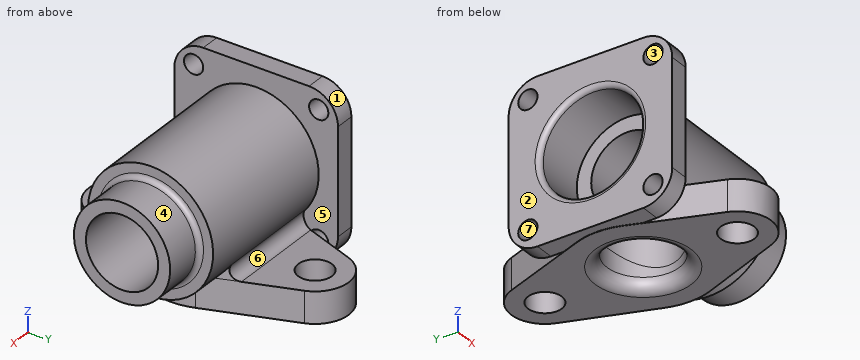
```python
from build123d import *

# Parameters (mm, degrees)
SKETCH1_R           = 7
SKETCH1_R_2         = 15
BOSS_EXTRUDE1_DEPTH = 13
SKETCH2_R           = 4
BOSS_EXTRUDE2_DEPTH = 4
SKETCH5_R           = 26
BOSS_EXTRUDE3_DEPTH = 63
FILLET6_R           = 4
FILLET7_R           = 4
SKETCH6_R           = 21
CUT_EXTRUDE1_DEPTH  = 22
CUT_EXTRUDE2_REACH  = 93.894
SKETCH7_R           = 15
BOSS_EXTRUDE4_START = -43
SKETCH9_R           = 15
BOSS_EXTRUDE4_DEPTH = 43
FILLET10_R          = 2
SKETCH12_R          = 20
BOSS_EXTRUDE5_DEPTH = 17
FILLET14_R          = 2
CUT_EXTRUDE4_REACH  = 119.421
SKETCH16_R          = 15
CUT_EXTRUDE5_REACH  = 106.103
SKETCH17_R          = 15
FILLET17_R          = 5


with BuildPart() as part:
    # Sketch1 → Boss-Extrude1 (new body)
    with BuildSketch(Plane.XY):
        with BuildLine():
            Line((-13.182592111, 45.551865312), (-26.129780791, 9.343289347))
            ThreePointArc((-26.129780791, 9.343289347), (-27.749182892, -0.212952692), (-25.983307196, -9.743215442))
            Line((-25.983307196, -9.743215442), (-13.108695522, -44.07736233))
            ThreePointArc((-13.108695522, -44.07736233), (0, -53.161866251), (13.108695522, -44.07736233))
            Line((13.108695522, -44.07736233), (25.983307196, -9.743215442))
            ThreePointArc((25.983307196, -9.743215442), (27.749182892, -0.212952692), (26.129780791, 9.343289347))
            Line((26.129780791, 9.343289347), (13.182592111, 45.551865312))
            ThreePointArc((13.182592111, 45.551865312), (0, 54.838133749), (-13.182592111, 45.551865312))
        make_face()
        with Locations((0, 40.838133749)):
            Circle(SKETCH1_R, mode=Mode.SUBTRACT)
        with Locations((0, -39.161866251)):
            Circle(SKETCH1_R, mode=Mode.SUBTRACT)
        Circle(SKETCH1_R_2, mode=Mode.SUBTRACT)
    extrude(amount=-BOSS_EXTRUDE1_DEPTH)



with BuildPart() as body_2:
    # Sketch2 → Boss-Extrude2 (new, symmetric)
    with BuildSketch(Plane(origin=(-27.5, 0, 0), x_dir=(0, 0, -1), z_dir=(1, 0, 0))):
        with BuildLine():
            Line((-43.103277086, 34), (0.896722914, 34))
            ThreePointArc((0.896722914, 34), (9.382004289, 30.485281374), (12.896722914, 22))
            Line((12.896722914, 22), (12.896722914, -22))
            ThreePointArc((12.896722914, -22), (9.382004289, -30.485281374), (0.896722914, -34))
            Line((0.896722914, -34), (-43.103277086, -34))
            ThreePointArc((-43.103277086, -34), (-51.58855846, -30.485281374), (-55.103277086, -22))
            Line((-55.103277086, -22), (-55.103277086, 22))
            ThreePointArc((-55.103277086, 22), (-51.58855846, 30.485281374), (-43.103277086, 34))
        make_face()
        with Locations((-47.103277086, 26)):
            Circle(SKETCH2_R, mode=Mode.SUBTRACT)
        with Locations((-47.103277086, -26)):
            Circle(SKETCH2_R, mode=Mode.SUBTRACT)
        with Locations((4.896722914, 26)):
            Circle(SKETCH2_R, mode=Mode.SUBTRACT)
        with Locations((4.896722914, -26)):
            Circle(SKETCH2_R, mode=Mode.SUBTRACT)
    extrude(amount=BOSS_EXTRUDE2_DEPTH, both=True)


with BuildPart() as part_1:
    add(part.part)

    add(body_2.part)  # Boss-Extrude3 merges body 2
    # Sketch5 → Boss-Extrude3 (add)
    with BuildSketch(Plane(origin=(-23.5, 0, 0), x_dir=(0, 0, -1), z_dir=(1, 0, 0))):
        with Locations(Location((-21.103277086, 0, 0), (0, 0, 324.258878137))):
            Circle(SKETCH5_R)
    extrude(amount=BOSS_EXTRUDE3_DEPTH)

    # Fillet6
    # the kernel refuses this fillet: 4 mm, written as the material it adds along each edge
    with BuildSketch(Plane(origin=(-47.149613866, -15.187221479, 0), x_dir=(0, -0.701013336910265, 0.7131481623575392), z_dir=(1, 0, 0))) as fillet6_piece_1_section:
        with BuildLine():
            CenterArc((9.484070542, 3.94221812), FILLET6_R, 135.491639194, 124.757843476)
            Line((6.631477893, 6.746271467), (0, 0))
            ThreePointArc((0, 0), (4.403318466, 0.375582222), (8.806636932, 0))
        make_face()
    fillet6_piece_1 = extrude(amount=94.74114261, mode=Mode.PRIVATE)
    fillet6_piece_1 = split(fillet6_piece_1, bisect_by=Plane(origin=(19.603312595, -26.757450692, 1.537679947), z_dir=(-0.9363353944532133, 0.35110686278417497, 0)), keep=Keep.TOP, mode=Mode.PRIVATE)
    fillet6_piece_1 = split(fillet6_piece_1, bisect_by=Plane(origin=(-19.602415947, -26.759841882, 1.537679947), z_dir=(0.9363353944532126, 0.35110686278417685, 0)), keep=Keep.TOP, mode=Mode.PRIVATE)
    add(fillet6_piece_1)

    # Fillet7
    # the kernel refuses this fillet: 4 mm, written as the material it adds along each edge
    with BuildSketch(Plane(origin=(47.689765613, 15.187221479, 0), x_dir=(0, 1, 0), z_dir=(-1, 0, 0))) as fillet7_piece_1_section:
        with BuildLine():
            CenterArc((9.459845546, -4), FILLET7_R, 90, 124.757843476)
            ThreePointArc((6.173569943, -6.280436945), (3.354630742, -2.876930326), (0, 0))
            Line((0, 0), (9.459845546, 0))
        make_face()
    fillet7_piece_1 = extrude(amount=94.839379478, mode=Mode.PRIVATE)
    fillet7_piece_1 = split(fillet7_piece_1, bisect_by=Plane(origin=(-19.975054308, 26.555819952, 1.538101515), z_dir=(0.941613722197052, -0.33669511159239174, 0)), keep=Keep.TOP, mode=Mode.PRIVATE)
    fillet7_piece_1 = split(fillet7_piece_1, bisect_by=Plane(origin=(19.97656332, 26.551599793, 1.538101515), z_dir=(-0.9416137221970524, -0.3366951115923907, 0)), keep=Keep.TOP, mode=Mode.PRIVATE)
    add(fillet7_piece_1)

    # Sketch6 → Cut-Extrude1 (cut)
    with BuildSketch(Plane.ZY.offset(31.5)):
        with Locations((21.103277086, 0)):
            Circle(SKETCH6_R)
    extrude(amount=-CUT_EXTRUDE1_DEPTH, mode=Mode.SUBTRACT)

    # Sketch7 → Cut-Extrude2 (cut, up to next)
    with BuildSketch(Plane.ZY.offset(9.5), mode=Mode.PRIVATE) as cut_extrude2_sk1:
        with Locations((21.103277086, 0)):
            Circle(SKETCH7_R)
    cut_extrude2_tool1 = extrude(cut_extrude2_sk1.sketch, amount=-CUT_EXTRUDE2_REACH, mode=Mode.PRIVATE) & part_1.part
    add(cut_extrude2_tool1.solids().sort_by_distance((-9.5, 0, 21.103277))[0], mode=Mode.SUBTRACT)

    # Sketch9 → Boss-Extrude4 (add)
    with BuildSketch(Plane(origin=(39.5, 0, 0), x_dir=(0, 0, -1), z_dir=(1, 0, 0)).offset(BOSS_EXTRUDE4_START)):
        with Locations(Location((-21.103277086, 0, 0), (0, 0, 180))):
            Circle(SKETCH9_R)
    extrude(amount=BOSS_EXTRUDE4_DEPTH)

    # Fillet10
    fillet10_edges = [part_1.edges().sort_by_distance(p)[0] for p in [
        (-31.5, 0, 0.103277086),
    ]]
    fillet(fillet10_edges, radius=FILLET10_R)

    # Sketch12 → Boss-Extrude5 (add)
    with BuildSketch(Plane(origin=(39.5, 0, 0), x_dir=(0, 0, -1), z_dir=(1, 0, 0))):
        with Locations((-21.103277086, 0)):
            Circle(SKETCH12_R)
    extrude(amount=BOSS_EXTRUDE5_DEPTH)

    # Fillet14
    fillet14_edges = [part_1.edges().sort_by_distance(p)[0] for p in [
        (39.5, 0, 41.103277086),
    ]]
    fillet(fillet14_edges, radius=FILLET14_R)

    # Sketch16 → Cut-Extrude4 (cut, up to next)
    with BuildSketch(Plane(origin=(56.5, 0, 0), x_dir=(0, 0, -1), z_dir=(1, 0, 0)), mode=Mode.PRIVATE) as cut_extrude4_sk1:
        with Locations(Location((-21.103277086, 0, 0), (0, 0, 180))):
            Circle(SKETCH16_R)
    cut_extrude4_tool1 = extrude(cut_extrude4_sk1.sketch, amount=-CUT_EXTRUDE4_REACH, mode=Mode.PRIVATE) & part_1.part
    add(cut_extrude4_tool1.solids().sort_by_distance((56.5, 0, 21.103277))[0], mode=Mode.SUBTRACT)

    # Sketch17 → Cut-Extrude5 (cut, up to next)
    with BuildSketch(Plane(origin=(0, 0, -13), x_dir=(-1, 0, 0), z_dir=(0, 0, -1)), mode=Mode.PRIVATE) as cut_extrude5_sk1:
        with Locations(Location((0, 0, 0), (0, 0, 180))):
            Circle(SKETCH17_R)
    cut_extrude5_tool1 = extrude(cut_extrude5_sk1.sketch, amount=-CUT_EXTRUDE5_REACH, mode=Mode.PRIVATE) & part_1.part
    add(cut_extrude5_tool1.solids().sort_by_distance((0, 0, -13))[0], mode=Mode.SUBTRACT)

    # Fillet17
    fillet17_edges = [part_1.edges().sort_by_distance(p)[0] for p in [
        (-15, 0, -13),
    ]]
    fillet(fillet17_edges, radius=FILLET17_R)


solid = part_1.part
```
For this review, take the finished solid that the model builds, in its own axes (mm). Face numbers are marked on the shaded views. A direction names the side the tool comes from. Coordinates: 2 decimals unless noted, no trailing zeros. Order: outer loops, then holes, each group sorted by start corner. A loop starts at its lowest first (then second) coordinate and runs counter-clockwise, first axis right, second up. Notation, with made-up numbers: (42, 67.25) - (101, 67.25) arc R21 cw to (101, 88.25) - close; hole circle Ø9 at (-9.75, 46.25). An arc over 180 degrees is marked (long way). Answer as a JSON object with one key per item and string values. Group by question number.
1. We need section A-A on y = 0. Give the number of separate pieces and of enclosed holes in the cut face, then the cut area to 3 significant figures.
2. The part is to be moulded in two halves that separate along Z. For the marked faces 1, 2, 3 and 4, say which applies: pulls with the +Z half, pulls with the -Z half, needs draft (parallel to the pull), parting line crosses it, or undercut.
3. We need section C-C on x = 0. State the section outline as (y, z) points, then the cut area to 3 significant figures.
4. For probe 1 along X at (y, z) = (0, -6); probe 2 along Z at (x, y) = (11, 27.5); probe 3 along X at (y, z) = (0, -4.25), list the stretches that pass through material, from the lowest coordinate up.
5. For the marked faces 5, 6 and 7, list the 3-axis set-ups (+Z, -Z, +X, -X, +Y, -Y) from which the entire face can be reached by the end or side of a thin tool; tool diameter is ignored.
6. We need section B-B on y = 28. State the section outline as (x, z) points.
7. Clearance check with flat-ended pins moving along their axes: P1, Ø8.5, axis at x = 0, y = 40.84, coming from the +Z side; P2, Ø14.5, axis at x = 9.5, y = -42, coming from the +Z side; P3, Ø10, axis at y = 6.5, z = 30, coming from the -X side; P4, Ø2.5, axis at x = -26.5, z = 26, coming from the -Y side. State where each tip first meets the part, or that it passes through.
Final values:
{
 "1": {"separate pieces": "3", "enclosed holes": "0", "area": "1,460 mm²"},
 "2": {"face 1": "pulls with the +Z half", "face 2": "needs draft", "face 3": "undercut", "face 4": "parting line crosses it"},
 "3": {"outline": "(-53.16, -13) - (-46.16, -13) - (-46.16, 0) - (-53.16, 0) - close; (-32.16, -13) - (-20, -13) arc R5 ccw to (-15, -8) - (-15, 21.1) arc R15 cw to (15, 21.1) - (15, -8) arc R5 ccw to (20, -13) - (33.84, -13) - (33.84, 0) - (24.65, 0) arc R4 cw to (21.36, 6.28) arc R26 ccw (long way) to (-21.36, 6.28) arc R4 cw to (-24.65, 0) - (-32.16, 0) - close; (47.84, -13) - (54.84, -13) - (54.84, 0) - (47.84, 0) - close", "area": "1,710 mm²"},
 "4": {"probe 1": "-31.5 to -15, 15 to 27.75", "probe 2": "-13 to 0", "probe 3": "-31.5 to -15, 15 to 39.5"},
 "5": {"face 5": "none", "face 6": "+X, +Y", "face 7": "-X"},
 "6": {"outline": "(-31.5, -11.29) - (-23.5, -11.29) - (-23.5, -8.36) - (-31.5, -8.36) - close; (-31.5, -1.43) - (-23.5, -1.43) - (-23.5, 43.64) - (-31.5, 43.64) - close; (-31.5, 50.57) - (-23.5, 50.57) - (-23.5, 53.5) - (-31.5, 53.5) - close; (-19.46, -13) - (19.46, -13) - (19.46, 0) - (-19.46, 0) - close"},
 "7": {"P1": "through", "P2": "z = 0", "P3": "x = -9.5", "P4": "y = -34"}
}
